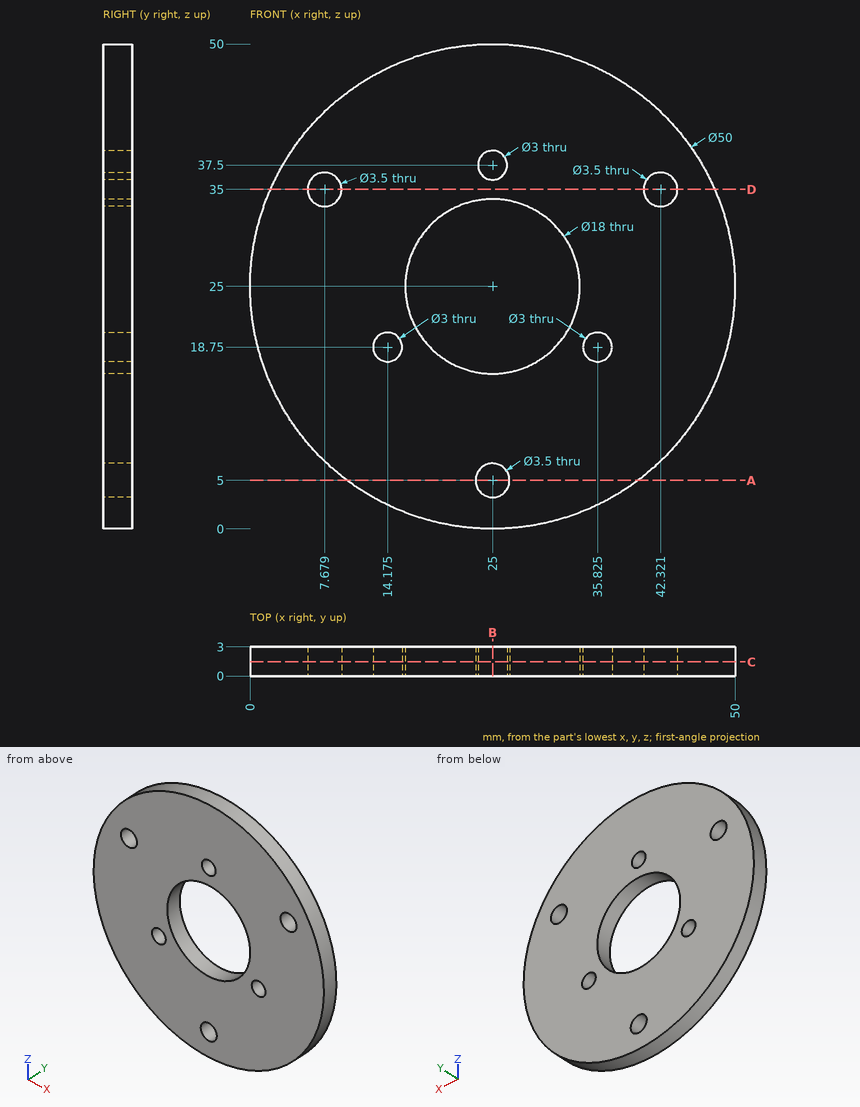
Part print with two shaded views. Sizes in mm from the minimum x, y, z corner. Round coordinates to 2 decimals unless told otherwise and drop trailing zeros. Loops run counter-clockwise (first coordinate to the right, second up) from the corner with the lowest first, then second, coordinate; pieces in that order, holes last. Notation, with made-up numbers: (-19.75, -5) - (28.25, -5) arc R15 cw to (28.25, 8) - close; hole circle Ø4 at (-2, -39). An arc over 180 degrees is marked (long way). Put each result on its own line as item: value.
1. Slice it at A-A on z = 5. List the corners of the cut face in (x, y).
Geometry check:
outline: (10, 0) - (23.25, 0) - (23.25, 3) - (10, 3) - close; (26.75, 0) - (40, 0) - (40, 3) - (26.75, 3) - close
2. Wall check: line 1 (X direction, y = 1.7, z = 36.5) (1 decimal); line 2 (X direction, y = 1.7, z = 18.75) (1 decimal); line 3 (X direction, y = 1.65, z = 35). Give the ranges that are in metal, low to high.
Geometry check:
line 1: 2.8 to 6.8, 8.6 to 23.9, 26.1 to 41.4, 43.2 to 47.2
line 2: 0.8 to 12.7, 15.7 to 18.5, 31.5 to 34.3, 37.3 to 49.2
line 3: 2.09 to 5.93, 9.43 to 40.57, 44.07 to 47.91
3. Slice it at B-B on x = 25. List the corners of the cut face in (y, z).
Geometry check:
outline: (0, 0) - (3, 0) - (3, 3.25) - (0, 3.25) - close; (0, 6.75) - (3, 6.75) - (3, 16) - (0, 16) - close; (0, 34) - (3, 34) - (3, 36) - (0, 36) - close; (0, 39) - (3, 39) - (3, 50) - (0, 50) - close
4. Slice it at D-D on z = 35. List the corners of the cut face in (x, y).
Geometry check:
outline: (2.09, 0) - (5.93, 0) - (5.93, 3) - (2.09, 3) - close; (9.43, 0) - (40.57, 0) - (40.57, 3) - (9.43, 3) - close; (44.07, 0) - (47.91, 0) - (47.91, 3) - (44.07, 3) - close
5. Pin check, flat tips, straight feed: P1, Ø16, axis at x = 25, z = 25, coming from the +Y side; P2, Ø1.5, axis at y = 1.5, z = 16, coming from the +X side; P3, Ø1.5, axis at x = 7, y = 1.5, coming from the +Z side (1 decimal). Stop position of each tip, or through.
Geometry check:
P1: through
P2: x = 48.6
P3: z = 43.1
6. Slice it at C-C on y = 1.45. Give the number of separate pieces and of enclosed holes in the cut face, and give its area (3 significant figures).
Geometry check:
separate pieces: 1
enclosed holes: 7
area: 1,660 mm²
